Read the model definition and answer for the solid it produces. Units are mm, in the model's axes. A direction names the side the tool comes from. Coordinates: 2 decimals unless noted, no trailing zeros. Loops run counter-clockwise (first coordinate to the right, second up) from the corner with the lowest first, then second, coordinate; pieces in that order, holes last. Notation, with made-up numbers: (-24, 28.5) -> (24, 28.5) arc R31 cw to (24, 55.5) -> close; hole circle Ø10 at (80.25, 1.5). An arc over 180 degrees is marked (long way). Answer as a JSON object with one key per item and string values. Group by question number.
1) Determine the mould class of faces 1 (the face through (69, 34, 0)), 2 (the face through (137.15, 64.99, 7.4)), 3 (the face through (135, 47, 9)) for opening direction Y: released by +Y, released by -Y, zero draft, split by the parting line, or undercut.
2) Which of the six approach directions +Z, -Z, +X, -X, +Y, -Y give full straight-line access (tool end or side, diameter ignored) to faces 4 (the face through (135, 20, 11)), 5 (the face through (69, 34, 15))?
3) Flat-ended cylindrical pins translate along their axes: P1, Ø5.5, axis at x = 137, z = 6.5, coming from the +Y side; P2, Ø0.9, axis at x = 134, z = 7.5, coming from the -Y side; P3, Ø2, axis at y = 21, z = 8, coming from the +X side. Find the tip coordinate at first contact, or state that the pin passes through.
4) Consider probe 1 along Z at (x, y) = (134.5, 22); probe 2 along Y at (x, z) = (132, 4.5); probe 3 along X at (y, z) = (34, 5.75). Determine where each line is inside the solid, lowest interval first. Write a range as [from, to].
5) Section A-A, the plane y = 20 is taken. Give the vertices of the cut face in (x, z), plus the area to 3 significant figures.
6) Section B-B, the plane x = 132 is taken. Give the vertices of the cut face in (y, z).
from build123d import *

# Parameters (mm, degrees)
Y_KSEKLIK_EKSTR_ZYON1_DEPTH = 15
IZIM2_W                     = 7
IZIM2_H                     = 10
IZIM2_W_2                   = 3
IZIM2_H_2                   = 7
KES_EKSTR_ZYON1_DEPTH       = 10


with BuildPart() as part:
    # Çizim1 → Yükseklik-Ekstrüzyon1 (new body)
    with BuildSketch(Plane.XY):
        with BuildLine():
            Line((10, 0), (130, 0))
            ThreePointArc((130, 0), (137.071067812, 2.928932188), (140, 10))
            Line((140, 10), (140, 58))
            ThreePointArc((140, 58), (137.071067812, 65.071067812), (130, 68))
            Line((130, 68), (10, 68))
            ThreePointArc((10, 68), (2.928932188, 65.071067812), (0, 58))
            Line((0, 58), (0, 10))
            ThreePointArc((0, 10), (2.928932188, 2.928932188), (10, 0))
        make_face()
    extrude(amount=Y_KSEKLIK_EKSTR_ZYON1_DEPTH)

    # Çizim2 → Kes-Ekstrüzyon1 (cut)
    with BuildSketch(Plane(origin=(140, 0, 0), x_dir=(0, 0, -1), z_dir=(1, 0, 0))):
        with Locations((-7.5, 20)):
            Rectangle(IZIM2_W, IZIM2_H)
        with Locations((-7.5, 35)):
            Rectangle(IZIM2_W, IZIM2_H)
        with Locations((-7.5, 47.5)):
            Rectangle(IZIM2_W_2, IZIM2_H_2)
    extrude(amount=-KES_EKSTR_ZYON1_DEPTH, mode=Mode.SUBTRACT)


solid = part.part
Determined:
{
 "1": {"face 1": "zero draft", "face 2": "released by +Y", "face 3": "undercut"},
 "2": {"face 4": "+X", "face 5": "+Z, +X, -X, +Y, -Y"},
 "3": {"P1": "y = 67.05", "P2": "y = 0.65", "P3": "x = 130"},
 "4": {"probe 1": "[0, 4], [11, 15]", "probe 2": "[0.2, 15], [25, 30], [40, 67.8]", "probe 3": "[0, 130]"},
 "5": {"outline": "(0, 0) -> (140, 0) -> (140, 4) -> (130, 4) -> (130, 11) -> (140, 11) -> (140, 15) -> (0, 15) -> close", "area": "2,030 mm²"},
 "6": {"outline": "(0.2, 0) -> (67.8, 0) -> (67.8, 15) -> (0.2, 15) -> close; hole (15, 4) -> (25, 4) -> (25, 11) -> (15, 11) -> close; hole (30, 4) -> (40, 4) -> (40, 11) -> (30, 11) -> close; hole (44, 6) -> (51, 6) -> (51, 9) -> (44, 9) -> close"}
}
